Autodesk Inventor part; units mm, degrees
ref_plane "YZ Plane" through (0, 0, 0) normal (1, 0, 0) x (0, 1, 0)
ref_plane "XZ Plane" through (0, 0, 0) normal (0, 1, 0) x (-1, 0, 0)
ref_plane "XY Plane" through (0, 0, 0) normal (0, 0, 1) x (1, 0, 0)
sketch "Sketch1" plane through (0, 0, 0) normal (0, 1, 0) x (-1, 0, 0)
  circle A0 centre (0, 0) radius 9
  dimension "d0" = 18
extrude "Extrusion1" add sketch "Sketch1" along normal blind 64
sketch "Sketch2" plane through (0, 64, 0) normal (0, 1, 0) x (1, 0, 0)
  circle A0 centre (0, 0) radius 9
  circle A1 centre (0, 0) radius 3
  dimension "d3" = 6
extrude "Extrusion2" add sketch "Sketch2" along normal blind 1 contours A1
chamfer "Chamfer1" distance 0.5 angle 45 1 edges at (-3, 65, 0)
fillet "Fillet1" radius 0.25 2 edges at (9, 64, 0) (9, 0, 0)
properties part number "18650" material "Steel"
Design review of the part built by this model. Coordinates are the model's own, in mm. A direction names the side the tool comes from. Round coordinates to 2 decimals unless told otherwise and drop trailing zeros. Write each loop counter-clockwise with the first axis right and the second up, starting at its lowest first coordinate (ties: lowest second). Pieces come first, ordered by that corner, then holes.
Item 1: Consider section A-A on y = 20. Give the boundary of the cut face in (x, z).
Item 2: For faces 1 (the cylindrical face through (-3, 64.2, 0.1)), 2 (the flat face through (0, 65, 0)), list the 3-axis set-ups (+Z, -Z, +X, -X, +Y, -Y) from which the entire face can be reached by the end or side of a thin tool; tool diameter is ignored.
Item 3: Wall thickness on L1, parallel to Y at x = -6.75, z = -0.75; L2, parallel to X at y = 6, z = 0.25; L3, parallel to Z at x = 1.5, y = 55.5: over which ranges is each line inside the solid? List them lowest first.
Item 4: For pin 1 Ø6 at (x, z) = (1.5, -5) entering from +Y; pin 2 Ø1.5 at (x, y) = (-2.5, 45) entering from -Z; pin 3 Ø2 at (y, z) = (47, 6) entering from -X; pin 4 Ø2 at (y, z) = (25.5, 2) entering from +X, all flat-tipped, find the tip position at first contact; note any pin that passes through.
Check values:
1. outline: circle Ø18 at (0, 0)
2. face 1: +Y
2. face 2: +Z, -Z, +X, -X, +Y
3. L1: y = 0 to 64
3. L2: x = -9 to 9
3. L3: z = -8.87 to 8.87
4. pin 1: stops at y = 65
4. pin 2: stops at z = -8.83
4. pin 3: stops at x = -7.48
4. pin 4: stops at x = 8.94
